from build123d import *

# Parameters (mm, degrees)
SKETCH1_W                 = 60
SKETCH1_H                 = 120
BOSS_EXTRUDE1_DEPTH       = 2
SKETCH2_R                 = 3.814375117
CUT_EXTRUDE1_DEPTH        = 2
F_4_CLEARANCE_HOLE2_D     = 3.2639
F_4_CLEARANCE_HOLE2_DEPTH = 10
F_4_CLEARANCE_HOLE2_TIP   = 0.980574487


with BuildPart() as part:
    # Sketch1 → Boss-Extrude1 (new body)
    with BuildSketch(Plane.XY):
        with Locations((0, 79.160593828)):
            Rectangle(SKETCH1_W, SKETCH1_H)
    extrude(amount=BOSS_EXTRUDE1_DEPTH)

    # Sketch2 → Cut-Extrude1 (cut)
    with BuildSketch(Plane(origin=(0, 0, 0), x_dir=(-1, 0, 0), z_dir=(0, 0, -1))):
        with Locations((0, 75.261)):
            Circle(SKETCH2_R)
    extrude(amount=-CUT_EXTRUDE1_DEPTH, mode=Mode.SUBTRACT)

    # #4 Clearance Hole2
    with Locations(Plane.XY.offset(2)):
        with Locations((0, 33.332), (0, 23.992)):
            Hole(F_4_CLEARANCE_HOLE2_D / 2, depth=F_4_CLEARANCE_HOLE2_DEPTH)
            with Locations((0, 0, -(F_4_CLEARANCE_HOLE2_DEPTH + F_4_CLEARANCE_HOLE2_TIP / 2))):  # 118° drill point
                Cone(0, F_4_CLEARANCE_HOLE2_D / 2, F_4_CLEARANCE_HOLE2_TIP, mode=Mode.SUBTRACT)


solid = part.part
Design review of the part built by this model. Coordinates are the model's own, in mm. Give positions to 0.01 mm unless a question says otherwise; leave off trailing zeros. Loops run counter-clockwise (first coordinate to the right, second up) from the corner with the lowest first, then second, coordinate; pieces in that order, holes last. Notation, with made-up numbers: M 10.5,-11.5 L 66.5,-11.5 A26 cw 66.5,26.5 Z; hole C -1.5,14 d3. An arc over 180 degrees is marked long. Write item = value, one per line.
Q1. We need section A-A (x = 0). Give the boundary of the cut face in (y, z).
Output values:
outline = M 19.16,0 L 22.36,0 L 22.36,2 L 19.16,2 Z; M 25.62,0 L 31.7,0 L 31.7,2 L 25.62,2 Z; M 34.96,0 L 71.45,0 L 71.45,2 L 34.96,2 Z; M 79.08,0 L 139.16,0 L 139.16,2 L 79.08,2 Z
Q2. Draft analysis for pull direction Y (two halves, no side actions). For faces 1 (the flat face through (0, 80, 2)), 2 (the cylindrical face through (-0.877, 34.708, 0.986)), 3 (the cylindrical face through (0.497, 79.043, 0.986)), state which applies: +Y half, -Y half, draft (parallel to the pull), parting line (faces both ways), or undercut.
Output values:
face_1 = draft
face_2 = undercut
face_3 = undercut
Q3. To check wall thickness, follow line 1 (Y direction, x = 0, z = 0.4); line 2 (X direction, y = 72, z = 1.45). State the ranges of each line that lie inside material, in increasing order. Write a range as [from, to].
Output values:
line_1 = [19.16, 22.36], [25.62, 31.7], [34.96, 71.45], [79.08, 139.16]
line_2 = [-30, -1.98], [1.98, 30]
